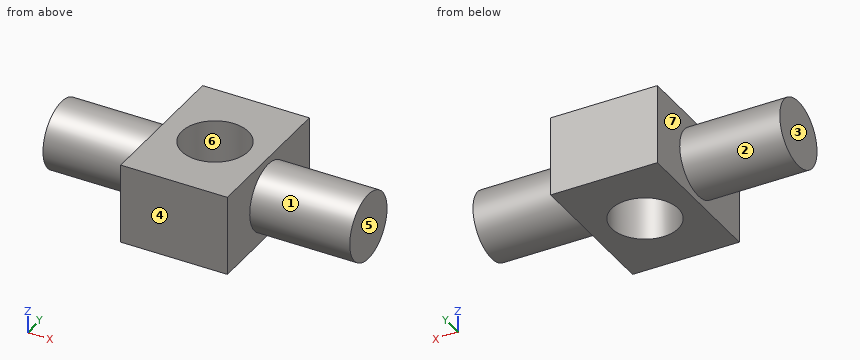
from build123d import *

# Parameters (mm, degrees)
SKETCH_1_W          = 16
SKETCH_1_H          = 22
EXTRUDE_1_DEPTH     = 6
SKETCH_2_R          = 5
EXTRUDE_2_DEPTH     = 15
SKETCH_3_R          = 5
CUT_EXTRUDE_1_DEPTH = 13


with BuildPart() as part:
    # 草图1 → 凸台-拉伸1 (new body, symmetric)
    with BuildSketch(Plane.XY):
        Rectangle(SKETCH_1_W, SKETCH_1_H)
    extrude(amount=EXTRUDE_1_DEPTH, both=True)

    # 草图2 → 凸台-拉伸2 (add)
    with BuildSketch(Plane(origin=(8, 0, 0), x_dir=(0, 0, -1), z_dir=(1, 0, 0))):
        Circle(SKETCH_2_R)
    extrude_2 = extrude(amount=EXTRUDE_2_DEPTH)

    # 镜向1: 凸台-拉伸2 across plane
    add(extrude_2.mirror(Plane(origin=(0, 0, 0), x_dir=(0, 0, 1), z_dir=(1, 0, 0))))

    # 草图3 → 切除-拉伸1 (cut, through all)
    with BuildSketch(Plane.XY.offset(6)):
        Circle(SKETCH_3_R)
    extrude(amount=-CUT_EXTRUDE_1_DEPTH, mode=Mode.SUBTRACT)


solid = part.part
Work out the finished part from the listing and answer in its coordinate system (mm). Face numbers are marked on the shaded views. A direction names the side the tool comes from. Give positions to 0.01 mm unless a question says otherwise; leave off trailing zeros. Loops run counter-clockwise (first coordinate to the right, second up) from the corner with the lowest first, then second, coordinate; pieces in that order, holes last. Notation, with made-up numbers: (3.5, 31.5) -> (24.5, 31.5) arc R11 cw to (24.5, 52.5) -> close; hole circle Ø5 at (74, 28.5). An arc over 180 degrees is marked (long way). Use a Markdown table: item, result. Add a question column.
1) For a pull along X with two mould halves and no side action, classify the marked faces 4, 5, 6 and 7 as +X half, -X half, draft (parallel to the pull), parting line (faces both ways), or undercut.
2) Which of the six approach directions +Z, -Z, +X, -X, +Y, -Y give full straight-line access (tool end or side, diameter ignored) to the marked faces 1, 2 and 3?
3) The part is cut by section A-A, the plane x = 0. Determine the outline of the cut face in (y, z), plus the area to 3 significant figures.
4) The part is cut by section B-B, the plane z = 0. Determine the outline of the cut face in (x, y), plus the area to 3 significant figures.
5) The part is cut by section D-D, the plane z = 3. Determine the outline of the cut face in (x, y).
6) Each of these flat-tipped pins is pushed along its axis until it touches: P1, Ø6, axis at x = -15, y = 8.5, coming from the +Z side; P2, Ø5, axis at y = 7.5, z = 1.5, coming from the +X side; P3, Ø6, axis at y = -7, z = -2.5, coming from the +X side; P4, Ø10, axis at x = -14.5, y = -1, coming from the +Z side. Where does it stop, or does it pass through?
7) Consider line 1 along Y through (x, z) = (0, -0.75); line 2 along Y through (x, z) = (-3, -4.75); line 3 along X through (y, z) = (-2, 4). Determine where each line is inside the solid, lowest interval first.
8) The part is cut by section C-C, the plane y = 0. Determine the outline of the cut face in (x, z).
Reported:
| question | item | result |
|---|---|---|
| 1 | face 4 | draft |
| 1 | face 5 | +X half |
| 1 | face 6 | undercut |
| 1 | face 7 | -X half |
| 2 | face 1 | +X |
| 2 | face 2 | -X |
| 2 | face 3 | +Z, -Z, -X, +Y, -Y |
| 3 | outline | (-11, -6) -> (-5, -6) -> (-5, 6) -> (-11, 6) -> close; (5, -6) -> (11, -6) -> (11, 6) -> (5, 6) -> close |
| 3 | area | 144 mm^2 |
| 4 | outline | (-23, -5) -> (-8, -5) -> (-8, -11) -> (8, -11) -> (8, -5) -> (23, -5) -> (23, 5) -> (8, 5) -> (8, 11) -> (-8, 11) -> (-8, 5) -> (-23, 5) -> close; hole circle Ø10 at (0, 0) |
| 4 | area | 573 mm^2 |
| 5 | outline | (-23, -4) -> (-8, -4) -> (-8, -11) -> (8, -11) -> (8, -4) -> (23, -4) -> (23, 4) -> (8, 4) -> (8, 11) -> (-8, 11) -> (-8, 4) -> (-23, 4) -> close; hole circle Ø10 at (0, 0) |
| 6 | P1 | passes through |
| 6 | P2 | stops at x = 8 |
| 6 | P3 | stops at x = 23 |
| 6 | P4 | stops at z = 5 |
| 7 | line 1 | y = -11 to -5, 5 to 11 |
| 7 | line 2 | y = -11 to -4, 4 to 11 |
| 7 | line 3 | x = -23 to -4.58, 4.58 to 23 |
| 8 | outline | (-23, -5) -> (-8, -5) -> (-8, -6) -> (-5, -6) -> (-5, 6) -> (-8, 6) -> (-8, 5) -> (-23, 5) -> close; (5, -6) -> (8, -6) -> (8, -5) -> (23, -5) -> (23, 5) -> (8, 5) -> (8, 6) -> (5, 6) -> close |
